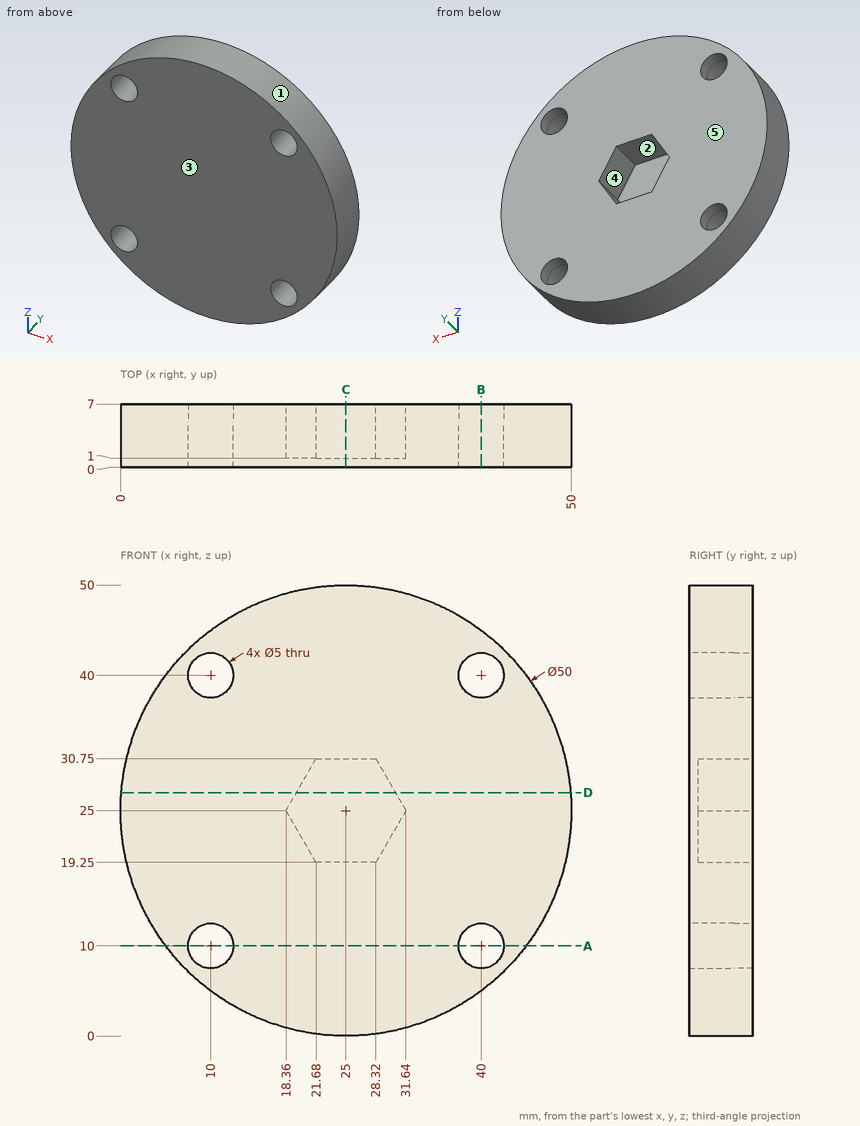
Geometry: see drawing. Coordinates: mm, zero at the bounding-box minimum. A direction names the side the tool comes from. Give positions to 0.01 mm unless a question says otherwise; leave off trailing zeros. Loops run counter-clockwise (first coordinate to the right, second up) from the corner with the lowest first, then second, coordinate; pieces in that order, holes last. Notation, with made-up numbers: (-12.5, -23) -> (-7.5, -23) arc R20 ccw to (-7.5, -9) -> close; hole circle Ø9 at (-18, 19). An arc over 180 degrees is marked (long way). Answer as a JSON object with one key per item and string values. Group by question number.
Item 1: Pull-direction query (Z, two-part tool) for the marked faces 1, 2 and 3; classes: released by +Z, released by -Z, zero draft, split by the parting line, or undercut.
Item 2: Cut plane D-D, the plane z = 27. Return the cut outline in (x, y) (1 decimal).
Item 3: Pin query (flat end, axial travel): P1, Ø3, axis at y = 3, z = 9, coming from the -X side (1 decimal); P2, Ø3, axis at y = 5.5, z = 37, coming from the +X side; P3, Ø4, axis at y = 2, z = 30, coming from the +X side; P4, Ø4, axis at x = 10, z = 40, coming from the -Y side. Return the tip coordinate at first contact, or that it passes through.
Item 4: Cut plane B-B, the plane x = 40. Return the cut outline in (y, z).
Item 5: Cut plane A-A, the plane z = 10. Return the cut outline in (x, y).
Item 6: Line query: probe 1 along X at (y, z) = (1.7, 10); probe 2 along X at (y, z) = (1.5, 11); probe 3 along Z at (x, y) = (22, 4.25). Output: solid intervals per line, ascending.
Item 7: Cut plane C-C, the plane x = 25. Return the cut outline in (y, z), and give its area (3 significant figures).
Item 8: Reachability of the marked faces 4 and 5 from +Z, -Z, +X, -X, +Y, -Y: full face, straight path, thin tool, end or side. Return the list, or none.
Checks:
{
 "1": {"face 1": "split by the parting line", "face 2": "undercut", "face 3": "zero draft"},
 "2": {"outline": "(0.1, 0) -> (49.9, 0) -> (49.9, 7) -> (30.5, 7) -> (30.5, 1) -> (19.5, 1) -> (19.5, 7) -> (0.1, 7) -> close"},
 "3": {"P1": "stops at x = 4.6", "P2": "stops at x = 47.69", "P3": "stops at x = 49.82", "P4": "passes through"},
 "4": {"outline": "(0, 5) -> (7, 5) -> (7, 7.5) -> (0, 7.5) -> close; (0, 12.5) -> (7, 12.5) -> (7, 37.5) -> (0, 37.5) -> close; (0, 42.5) -> (7, 42.5) -> (7, 45) -> (0, 45) -> close"},
 "5": {"outline": "(5, 0) -> (7.5, 0) -> (7.5, 7) -> (5, 7) -> close; (12.5, 0) -> (37.5, 0) -> (37.5, 7) -> (12.5, 7) -> close; (42.5, 0) -> (45, 0) -> (45, 7) -> (42.5, 7) -> close"},
 "6": {"probe 1": "x = 5 to 7.5, 12.5 to 37.5, 42.5 to 45", "probe 2": "x = 4.29 to 7.71, 12.29 to 37.71, 42.29 to 45.71", "probe 3": "z = 0.18 to 19.25, 30.75 to 49.82"},
 "7": {"outline": "(0, 0) -> (7, 0) -> (7, 19.25) -> (1, 19.25) -> (1, 30.75) -> (7, 30.75) -> (7, 50) -> (0, 50) -> close", "area": "281 mm²"},
 "8": {"face 4": "+Y", "face 5": "+Z, -Z, +X, -X, +Y"}
}
